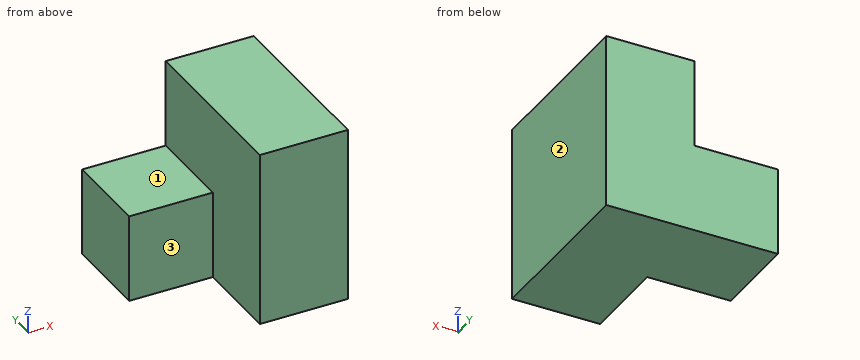
```python
from build123d import *

# Parameters (mm, degrees)
F1_W     = 25.4
F1_H     = 25.4
F2_DEPTH = 25.4
F0_W     = 25.4
F0_H     = 50.8
F3_DEPTH = 50.8
F7_DEPTH = 25.4
F5_W     = 25.4
F5_H     = 50.8
F8_DEPTH = 50.8


with BuildPart() as f2:
    # F1 (on Right) → F2 (new body)
    with BuildSketch(Plane.YZ):
        with Locations((-12.7, 15.4623677161)):
            Rectangle(F1_W, F1_H)
    extrude(amount=F2_DEPTH)


with BuildPart() as f3:
    # F0 (on Front) → F3 (new body)
    with BuildSketch(Plane.XZ):
        with Locations((-18.8699130297, 27.4796054423)):
            Rectangle(F0_W, F0_H)
    extrude(amount=F3_DEPTH)


with BuildPart() as f7:
    # F6 (on Front) → F7 (new body)
    with BuildSketch(Plane.XZ):
        Polygon((-49.5253019035, 0), (-24.1253019035, 0), (-23.6774347723, 25.4), (-49.5253019035, 25.4), align=None)
    extrude(amount=F7_DEPTH)

    # F5 (on Front) → F8 (join)
    with BuildSketch(Plane.XZ):
        with Locations((-12.7, 25.4)):
            Rectangle(F5_W, F5_H)
    extrude(amount=F8_DEPTH)


solid = f7.part
```
For this review, take the finished solid that the model builds, in its own axes (mm). Face numbers are marked on the shaded views. A direction names the side the tool comes from. Coordinates: 2 decimals unless noted, no trailing zeros. Loops run counter-clockwise (first coordinate to the right, second up) from the corner with the lowest first, then second, coordinate; pieces in that order, holes last. Notation, with made-up numbers: (-3, -36) - (44, -36) arc R10 ccw to (44, -26) - close; hole circle Ø3 at (75.25, 72.5). An arc over 180 degrees is marked (long way). Use one line per item in the form item = value. Start each with the question number.
1) Take a section at C-C (x = -43.5). State the section outline as (y, z) points, plus the area to 3 significant figures.
2) Take a section at D-D (y = -29.5). State the section outline as (x, z) points, plus the area to 3 significant figures.
3) Take a section at B-B (y = -10.5). State the section outline as (x, z) points, plus the area to 3 significant figures.
4) To check wall thickness, follow probe 1 along Y at (x, z) = (-36.5, 22.5); probe 2 along Z at (x, y) = (-33, -24). State the ranges of each line that lie inside material, in increasing order. Write a range as from..to.
5) Take a section at A-A (z = 13). State the section outline as (x, y) points, plus the area to 3 significant figures.
6) For pin 1 (12 mm diameter, centred on x = -42, z = 11, fed in from -Y); pin 2 (6 mm diameter, centred on x = -37, y = -11.5, fed in from +Z), all flat-tipped, find the tip position at first contact; note any pin that passes through.
7) For the marked faces 1, 2 and 3, list the 3-axis set-ups (+Z, -Z, +X, -X, +Y, -Y) from which the entire face can be reached by the end or side of a thin tool; tool diameter is ignored.
From the geometry:
q1.outline = (-25.4, 0) - (0, 0) - (0, 25.4) - (-25.4, 25.4) - close
q1.area = 645 mm2
q2.outline = (-25.4, 0) - (0, 0) - (0, 50.8) - (-25.4, 50.8) - close
q2.area = 1,290 mm2
q3.outline = (-49.53, 0) - (0, 0) - (0, 50.8) - (-25.4, 50.8) - (-25.4, 25.4) - (-49.53, 25.4) - close
q3.area = 1,900 mm2
q4.probe_1 = -25.4..0
q4.probe_2 = 0..25.4
q5.outline = (-49.53, -25.4) - (-25.4, -25.4) - (-25.4, -50.8) - (0, -50.8) - (0, 0) - (-49.53, 0) - close
q5.area = 1,900 mm2
q6.pin_1 = -25.4
q6.pin_2 = 25.4
q7.face_1 = +Z, -X, +Y, -Y
q7.face_2 = +Z, -Z, +X, +Y, -Y
q7.face_3 = +Z, -Z, -X, -Y
